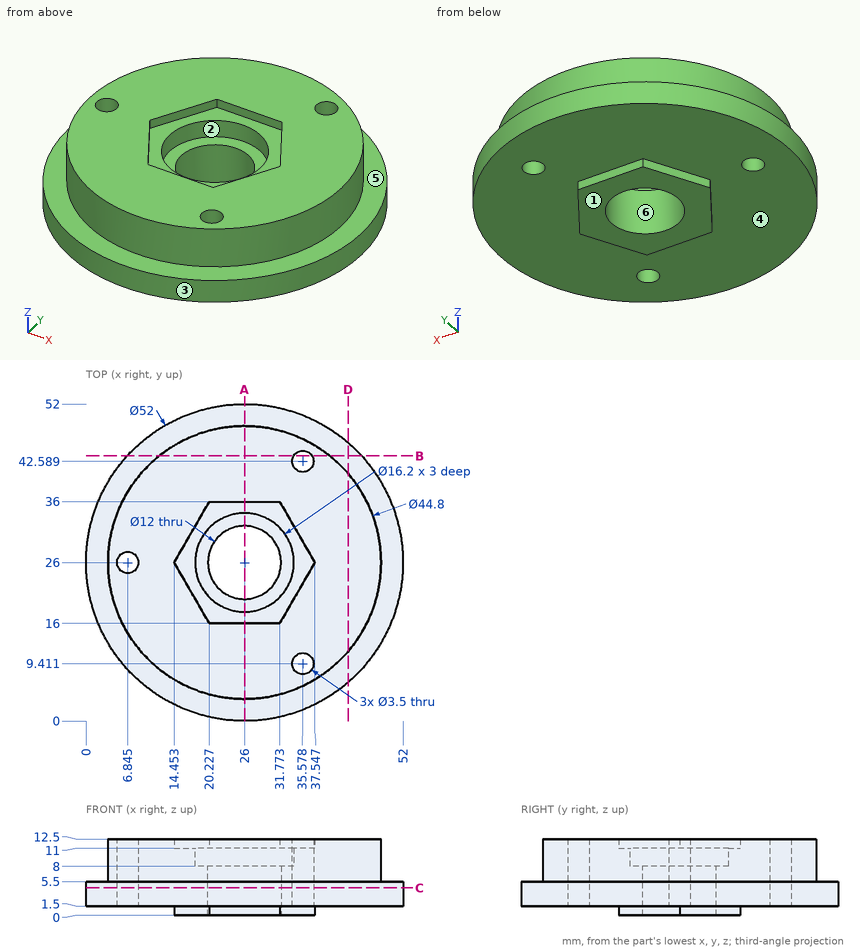
Answer from the drawing. Dimensions are ordinates in mm from the lowest x, y and z of the part. A direction names the side the tool comes from. Coordinates: 2 decimals unless noted, no trailing zeros. Write each loop counter-clockwise with the first axis right and the second up, starting at its lowest first coordinate (ties: lowest second). Pieces come first, ordered by that corner, then holes. Notation, with made-up numbers: (53.25, 82.5) - (97.25, 82.5) arc R11 ccw to (97.25, 95.5) - close; hole circle Ø7 at (3.25, 89). An arc over 180 degrees is marked (long way). Return JSON: item names as keys, results as strings. Group by question number.
Q1. Find the intervals of material crossed by line 1 along Y through (x, z) = (26, 12.25); line 2 along Y through (x, z) = (26, 9.4); line 3 along Z through (x, y) = (19.5, 27.5), in increasing order. Write a range as [from, to].
Q2. For a pull along Y with two mould halves and no side action, classify the marked faces 1, 2 and 3 as +Y half, -Y half, draft (parallel to the pull), parting line (faces both ways), or undercut.
Q3. The part is cut by section C-C on z = 4.5. State how many separate pieces and enclosed holes the cut face has, and give its area (3 significant figures).
Q4. The part is cut by section A-A on x = 26. Write down the section's boundary in (y, z), and give its area (3 significant figures).
Q5. Which of the six approach directions +Z, -Z, +X, -X, +Y, -Y give full straight-line access (tool end or side, diameter ignored) to the marked faces 4, 5 and 6?
Q6. The part is cut by section D-D on x = 43. Write down the section's boundary in (y, z).
Q7. The part is cut by section B-B on y = 43.5. Write down the section's boundary in (x, z), and give its area (3 significant figures).
Q8. Flat-ended cylindrical pins translate along their axes: pin 1 Ø4 at (x, y) = (35.58, 9.41) entering from -Z; pin 2 Ø5 at (y, z) = (44.5, 1.5) entering from +X (1 decimal); pin 3 Ø1.5 at (x, z) = (22, 9) entering from -Y. Find the tip coordinate at first contact, or state that the pin passes through.
Evaluation:
{
 "1": {"line 1": "y = [3.6, 16], [36, 48.4]", "line 2": "y = [3.6, 17.9], [34.1, 48.4]", "line 3": "z = [0, 8]"},
 "2": {"face 1": "draft", "face 2": "undercut", "face 3": "parting line"},
 "3": {"separate pieces": "1", "enclosed holes": "4", "area": "1,980 mm2"},
 "4": {"outline": "(0, 1.5) - (16, 1.5) - (16, 0) - (20, 0) - (20, 8) - (17.9, 8) - (17.9, 11) - (16, 11) - (16, 12.5) - (3.6, 12.5) - (3.6, 5.5) - (0, 5.5) - close; (32, 0) - (36, 0) - (36, 1.5) - (52, 1.5) - (52, 5.5) - (48.4, 5.5) - (48.4, 12.5) - (36, 12.5) - (36, 11) - (34.1, 11) - (34.1, 8) - (32, 8) - close", "area": "377 mm2"},
 "5": {"face 4": "-Z", "face 5": "+Z", "face 6": "+Z, -Z"},
 "6": {"outline": "(6.33, 1.5) - (45.67, 1.5) - (45.67, 5.5) - (40.59, 5.5) - (40.59, 12.5) - (11.41, 12.5) - (11.41, 5.5) - (6.33, 5.5) - close"},
 "7": {"outline": "(6.77, 1.5) - (34.08, 1.5) - (34.08, 12.5) - (12.02, 12.5) - (12.02, 5.5) - (6.77, 5.5) - close; (37.07, 1.5) - (45.23, 1.5) - (45.23, 5.5) - (39.98, 5.5) - (39.98, 12.5) - (37.07, 12.5) - close", "area": "317 mm2"},
 "8": {"pin 1": "stops at z = 1.5", "pin 2": "stops at x = 46.5", "pin 3": "stops at y = 3.84"}
}
